Here's how the part is built. I have some questions about the finished solid (model axes, mm). Coordinates: 2 decimals unless noted, no trailing zeros. Write each loop counter-clockwise with the first axis right and the second up, starting at its lowest first coordinate (ties: lowest second). Pieces come first, ordered by that corner, then holes. Notation, with made-up numbers: (-7, 44) -> (10, 44) arc R23 cw to (10, 82) -> close; hole circle Ø7 at (68, -38). An arc over 180 degrees is marked (long way). Use a Markdown table: item, result. Add a question column.
Item 1: Imagine slicing it at B-B, the plane y = 0. Write out the boundary of the cut face in (x, z), and give its area (3 significant figures).
Item 2: Imagine slicing it at A-A, the plane x = 0. Write out the boundary of the cut face in (y, z), and give its area (3 significant figures).
Item 3: Will these pins go through, and if not, where does the flat tip stop? pin 1 Ø1.6 at (x, y) = (-0.5, 0.5) entering from -Z; pin 2 Ø2 at (y, z) = (-2, 37.5) entering from +X; pin 3 Ø3 at (x, z) = (0.5, 28.5) entering from -Y.
Item 4: Imagine slicing it at D-D, the plane z = 16.5. Write out the boundary of the cut face in (x, y).
Item 5: If I drill on line 1 along Y through (x, z) = (0, -4.4); line 2 along Z through (x, y) = (-2.75, 0); line 3 along Y through (x, z) = (0, 40.5), over which ranges is the centre line in solid material (lowest first)? Write a range as from..to.
Item 6: Imagine slicing it at C-C, the plane z = 44. Write out the boundary of the cut face in (x, y).
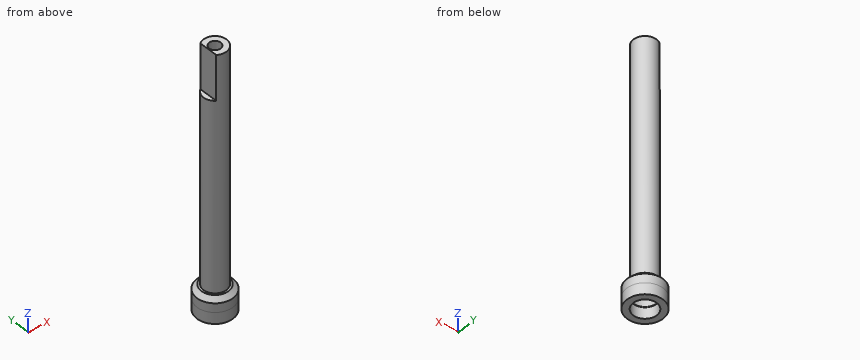
```python
from build123d import *

# Parameters (mm, degrees)
SKETCH_1_R          = 2.55
SKETCH_1_R_2        = 1.25
EXTRUDE_1_DEPTH     = 52
EXTRUDE_START       = 3
SKETCH_2_R          = 4
SKETCH_2_R_2        = 1.25
EXTRUDE_2_DEPTH     = 3
CUT_EXTRUDE_START   = -10
CUT_EXTRUDE_2_DEPTH = 10
EXTRUDE_START_2     = 2.5
SKETCH_9_R          = 4
SKETCH_9_R_2        = 2.6
EXTRUDE_3_DEPTH     = 2.5


with BuildPart() as part:
    # 草图1 → 凸台-拉伸1 (new body)
    with BuildSketch(Plane.XY):
        with Locations(Location((0, 0, 0), (0, 0, 180))):
            Circle(SKETCH_1_R)
        with Locations(Location((0, 0, 0), (0, 0, 180))):
            Circle(SKETCH_1_R_2, mode=Mode.SUBTRACT)
    extrude(amount=EXTRUDE_1_DEPTH)

    # 草图2 → 凸台-拉伸2 (add)
    with BuildSketch(Plane(origin=(0, 0, 0), x_dir=(-1, 0, 0), z_dir=(0, 0, -1)).offset(EXTRUDE_START)):
        Circle(SKETCH_2_R)
        Circle(SKETCH_2_R_2, mode=Mode.SUBTRACT)
    extrude(amount=-EXTRUDE_2_DEPTH)

    # 草图4 → 切除-拉伸2 (cut)
    with BuildSketch(Plane.XY.offset(52).offset(CUT_EXTRUDE_START)):
        with BuildLine():
            Line((-1.5, -2.062159063), (-1.5, 2.062159063))
            ThreePointArc((-1.5, 2.062159063), (-2.55, 0), (-1.5, -2.062159063))
        make_face()
    extrude(amount=CUT_EXTRUDE_2_DEPTH, mode=Mode.SUBTRACT)

    # 草图6 → 切除-旋转1 (revolve, cut)
    with BuildSketch(Plane(origin=(0, 0, 0), x_dir=(1, 0, 0), z_dir=(0, 1, 0)), mode=Mode.PRIVATE) as cut_revolve_1_sk:
        Polygon((0, 1.2), (2.2, 1.2), (2.5, 3), (0, 3), align=None)
    revolve(cut_revolve_1_sk.sketch.rotate(Axis((0, 0, -3), (0, 0, 1)), 180), axis=Axis((0, 0, -3), (0, 0, 1)), mode=Mode.SUBTRACT)

    # 草图8 → 切除-旋转3 (revolve, cut)
    with BuildSketch(Plane(origin=(0, 0, 0), x_dir=(1, 0, 0), z_dir=(0, 1, 0))):
        Polygon((4, 1), (3, 0), (4, 0), align=None)
    revolve(axis=Axis((0, 0, 0), (0, 0, -1)), mode=Mode.SUBTRACT)

    # 草图9 → 凸台-拉伸3 (add)
    with BuildSketch(Plane(origin=(0, 0, -3), x_dir=(-1, 0, 0), z_dir=(0, 0, -1)).offset(EXTRUDE_START_2)):
        with Locations(Location((0, 0, 0), (0, 0, 180))):
            Circle(SKETCH_9_R)
        Circle(SKETCH_9_R_2, mode=Mode.SUBTRACT)
    extrude(amount=-EXTRUDE_3_DEPTH)


solid = part.part
```
Ans:
| question | item | result |
|---|---|---|
| 1 | outline | (-4, -5.5) -> (-2.6, -5.5) -> (-2.6, -3) -> (-2.5, -3) -> (-2.2, -1.2) -> (-1.25, -1.2) -> (-1.25, 52) -> (-1.5, 52) -> (-1.5, 42) -> (-2.55, 42) -> (-2.55, 0) -> (-3, 0) -> (-4, -1) -> close; (1.25, -1.2) -> (2.2, -1.2) -> (2.5, -3) -> (2.6, -3) -> (2.6, -5.5) -> (4, -5.5) -> (4, -1) -> (3, 0) -> (2.55, 0) -> (2.55, 52) -> (1.25, 52) -> close |
| 1 | area | 143 mm^2 |
| 2 | outline | (-4, -5.5) -> (-2.6, -5.5) -> (-2.6, -3) -> (-2.5, -3) -> (-2.2, -1.2) -> (-1.25, -1.2) -> (-1.25, 52) -> (-2.55, 52) -> (-2.55, 0) -> (-3, 0) -> (-4, -1) -> close; (1.25, -1.2) -> (2.2, -1.2) -> (2.5, -3) -> (2.6, -3) -> (2.6, -5.5) -> (4, -5.5) -> (4, -1) -> (3, 0) -> (2.55, 0) -> (2.55, 52) -> (1.25, 52) -> close |
| 2 | area | 154 mm^2 |
| 3 | pin 1 | stops at z = -1.2 |
| 3 | pin 2 | stops at x = 2.35 |
| 3 | pin 3 | stops at y = -2.55 |
| 4 | outline | circle Ø5.1 at (0, 0); hole circle Ø2.5 at (0, 0) |
| 5 | line 1 | y = -4..-2.6, 2.6..4 |
| 5 | line 2 | z = -5.5..0 |
| 5 | line 3 | y = -2.55..-1.25, 1.25..2.55 |
| 6 | outline | (-1.5, -2.06) arc R2.55 ccw (long way) to (-1.5, 2.06) -> close; hole circle Ø2.5 at (0, 0) |
